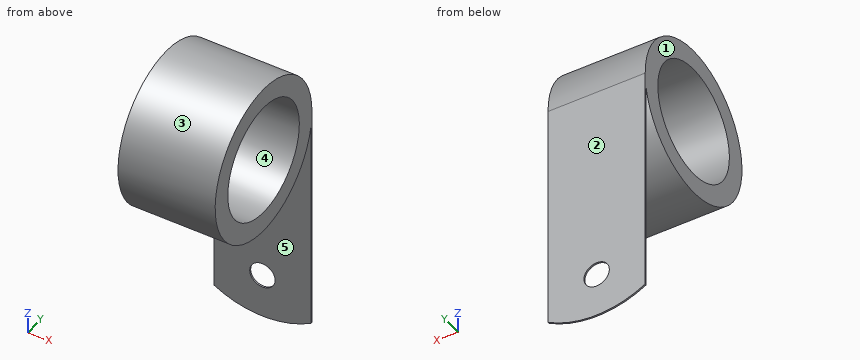
```python
from build123d import *

# Parameters (mm, degrees)
SKETCH1_R           = 11.176
BOSS_EXTRUDE1_DEPTH = 9.525
ONEHOLE_START       = -0.3048
SKETCH2_R           = 2.4892
ONEHOLE_DEPTH       = 0.3048


with BuildPart() as part:
    # Sketch1 → Boss-Extrude1 (new, symmetric)
    with BuildSketch(Plane(origin=(0, 0, 0), x_dir=(0, 0, -1), z_dir=(1, 0, 0))):
        with BuildLine():
            Line((0, 15.113), (47.625, 15.113))
            Line((47.625, 15.113), (47.625, 14.8082))
            Line((47.625, 14.8082), (3.019930754, 14.8082))
            ThreePointArc((3.019930754, 14.8082), (-1.517636715, -15.036606924), (0, 15.113))
        make_face()
        with Locations(Location((0, 0, 0), (0, 0, 180))):
            Circle(SKETCH1_R, mode=Mode.SUBTRACT)
    extrude(amount=BOSS_EXTRUDE1_DEPTH, both=True)

    # Sketch2 → OneHole (cut)
    with BuildSketch(Plane(origin=(0, 15.113, 0), x_dir=(1, 0, 0), z_dir=(0, 1, 0)).offset(ONEHOLE_START)):
        with Locations(Location((0, 38.9128, 0), (0, 0, 270))):
            Circle(SKETCH2_R)
        with BuildLine():
            Line((-9.525, 45.072783942), (-9.525, 48.26))
            Line((-9.525, 48.26), (9.525, 48.26))
            Line((9.525, 48.26), (9.525, 45.072783942))
            ThreePointArc((9.525, 45.072783942), (0, 47.625), (-9.525, 45.072783942))
        make_face()
    extrude(amount=ONEHOLE_DEPTH, mode=Mode.SUBTRACT)


solid = part.part
```
Geometry check sheet. Reference: the model listing, model coordinates, mm. Face numbers are marked on the shaded views. A direction names the side the tool comes from. Coordinates: 2 decimals unless noted, no trailing zeros. Order: outer loops, then holes, each group sorted by start corner. A loop starts at its lowest first (then second) coordinate and runs counter-clockwise, first axis right, second up.
Item 1: Section check A-A (x = 0). Enter the section's corners in (y, z) (3 decimals), plus the area to 3 significant figures.
Item 2: Section check D-D (x = 4.75). Enter the section's corners in (y, z).
Item 3: Tool access check on the marked faces 4 and 5. Record the directions out of +Z, -Z, +X, -X, +Y, -Y that give a thin tool (end or side, any length) a straight path to the whole face; none if there is none.
Item 4: Depth check by flat-ended pin: pin 1 (12 mm diameter, centred on y = -1.5, z = -22.5, fed in from -X); pin 2 (1 mm diameter, centred on x = 3.5, y = -8, fed in from +Z); pin 3 (5.5 mm diameter, centred on x = -3, z = -25, fed in from -Y); pin 4 (10 mm diameter, centred on x = -6.5, y = -1.5, fed in from -Z). Enter the tip coordinate at first touch or a pass-through.
Item 5: Mould release check, pull along Y, two halves, no side actions. Record for the marked faces 1, 2 and 3: released by +Y, released by -Y, zero draft, split by the parting line, or undercut.
Item 6: Section check C-C (z = -38). Enter the section's corners in (x, y) (3 decimals), plus the area to 3 significant figures.
Item 7: Section check B-B (y = 0). Enter the section's corners in (x, z) (3 decimals).
Item 8: Scan lines: line 1 along Y through (x, z) = (-5.5, -7.5); line 2 along Y through (x, z) = (-6.75, -39); line 3 along Y through (x, z) = (-5.5, 9.5). Record each from-to range of solid material in increasing order.
Check sheet entries:
1. outline: (14.808, -47.625) - (15.113, -47.625) - (15.113, -41.402) - (14.808, -41.402) - close; (14.808, -36.424) - (15.113, -36.424) - (15.113, 0) arc R15.113 ccw (long way) to (14.808, -3.02) - close; hole circle Ø22.352 at (0, 0)
1. area: 338 mm2
2. outline: (14.81, -47.02) - (15.11, -47.02) - (15.11, 0) arc R15.11 ccw (long way) to (14.81, -3.02) - close; hole circle Ø22.35 at (0, 0)
3. face 4: +X, -X
3. face 5: -Z, +X, -X
4. pin 1: passes through
4. pin 2: stops at z = 13.12
4. pin 3: stops at y = 14.81
4. pin 4: stops at z = -15.11
5. face 1: zero draft
5. face 2: released by +Y
5. face 3: undercut
6. outline: (-9.525, 14.808) - (-2.316, 14.808) - (-2.316, 15.113) - (-9.525, 15.113) - close; (2.316, 14.808) - (9.525, 14.808) - (9.525, 15.113) - (2.316, 15.113) - close
6. area: 4.39 mm2
7. outline: (-9.525, -15.113) - (9.525, -15.113) - (9.525, -11.176) - (-9.525, -11.176) - close; (-9.525, 11.176) - (9.525, 11.176) - (9.525, 15.113) - (-9.525, 15.113) - close
8. line 1: y = -13.12 to -8.29, 8.29 to 13.12, 14.81 to 15.11
8. line 2: y = 14.81 to 15.11
8. line 3: y = -11.75 to -5.89, 5.89 to 11.75
